CAD build for the part. Positions are in the model's coordinates, mm. A direction names the side the tool comes from. Coordinates: 2 decimals unless noted, no trailing zeros. Write each loop counter-clockwise with the first axis right and the second up, starting at its lowest first coordinate (ties: lowest second). Pieces come first, ordered by that corner, then holes. Notation, with made-up numbers: (64, 56.5) - (118, 56.5) arc R33 cw to (118, 91.5) - close; hole circle Ø1 at (-19.75, -8). An arc over 180 degrees is marked (long way). Answer in a Markdown table with one row per item. Add a question column.
Q1. Drill centre lines: line 1 along X through (y, z) = (21.5, -27); line 2 along Y through (x, z) = (36.5, 6.5); line 3 along Z through (x, y) = (14, 41). Where is each one in solid material? Low to high. Write a range as from..to.
Q2. Band-saw the part on B-B (y = 4.5). List the corners of the cut face in (x, z).
Q3. Band-saw the part on A-A (z = 5). List the corners of the cut face in (x, y).
Q4. Two-plate mould, pull along Z, no slides. Class faces 5 (the flat face through (-37.607, 3, 3)), 6 (the flat face through (0, 21, -43)), 7 (the flat face through (37.393, 21, -17)): +Z half, -Z half, draft (parallel to the pull), parting line (faces both ways), or undercut.
Q5. Band-saw the part on C-C (z = -4). List the corners of the cut face in (x, y), and give its area (3 significant figures).
Q6. Pin check, flat tips, straight feed: pin 1 (1 mm diameter, centred on y = 32.5, z = -13, fed in from -X); pin 2 (1.6 mm diameter, centred on x = -36.5, y = 40.5, fed in from +Z); pin 3 (1.6 mm diameter, centred on x = 36, z = -8, fed in from +Y). Stop position of each tip, or through.
Q7. Band-saw the part on D-D (x = 4.5). List the corners of the cut face in (y, z).
Q8. 3-axis set-ups, long thin cutter, end or side, ignore diameter. For faces 1 (the flat face through (35.393, 21, -18)), 2 (the flat face through (-37, 40, -9.5)), 3 (the flat face through (38, 6, 2)), 4 (the flat face through (-37, 43.5, -3)): which of +Z, -Z, +X, -X, +Y, -Y reach the whole face in a straight line?
```python
from build123d import *

# Parameters (mm, degrees)
BOSS_EXTRUDE1_DEPTH = 43.5
FILLET1_R           = 8
FILLET2_R           = 10
SKETCH3_W           = 3.5
SKETCH3_H           = 6
CUT_EXTRUDE1_DEPTH  = 57.75
BOSS_EXTRUDE2_DEPTH = 6


with BuildPart() as part:
    # Sketch2 → Boss-Extrude1 (new body)
    with BuildSketch(Plane(origin=(0, 0, 0), x_dir=(1, 0, 0), z_dir=(0, 1, 0))):
        Polygon((35.39315693, 0), (37.39315693, 0), (37.39315693, 45), (-37.60684307, 45), (-37.60684307, 0), (-35.60684307, 0), (-35.60684307, 43), (35.39315693, 43), align=None)
    extrude(amount=BOSS_EXTRUDE1_DEPTH)

    # Fillet1
    fillet1_edges = [part.edges().sort_by_distance(p)[0] for p in [
        (35.39315693, 21.75, -43),
        (-35.60684307, 21.75, -43),
    ]]
    fillet(fillet1_edges, radius=FILLET1_R)

    # Fillet2
    fillet2_edges = [part.edges().sort_by_distance(p)[0] for p in [
        (-37.60684307, 21.75, -45),
        (37.39315693, 21.75, -45),
    ]]
    fillet(fillet2_edges, radius=FILLET2_R)

    # Sketch3 → Cut-Extrude1 (cut, symmetric)
    with BuildSketch(Plane(origin=(0, 0, 0), x_dir=(0, 0, -1), z_dir=(1, 0, 0))):
        with Locations((7.75, 40.5)):
            Rectangle(SKETCH3_W, SKETCH3_H)
    extrude(amount=CUT_EXTRUDE1_DEPTH, both=True, mode=Mode.SUBTRACT)

    # Sketch4 → Boss-Extrude2 (add)
    with BuildSketch(Plane.XZ):
        Polygon((-37.60684307, -7), (-37.60684307, 6), (-35.60684307, 6), (-35.60684307, 7), (-37.60684307, 9), (-39.60684307, 9), (-39.60684307, -7), (-37.60684307, -9.5), align=None)
        Polygon((37.39315693, -7), (37.39315693, 6), (35.39315693, 6), (35.39315693, 7), (37.39315693, 9), (39.39315693, 9), (39.39315693, -7), (37.39315693, -9.5), align=None)
    extrude(amount=-BOSS_EXTRUDE2_DEPTH)


solid = part.part
```
Checked values:
| question | item | result |
|---|---|---|
| 1 | line 1 | x = -37.61..-35.61, 35.39..37.39 |
| 1 | line 2 | y = 0..6 |
| 1 | line 3 | z = -45..-43 |
| 2 | outline | (-39.61, -7) - (-37.61, -9.5) - (-37.61, -35) arc R10 ccw to (-27.61, -45) - (27.39, -45) arc R10 ccw to (37.39, -35) - (37.39, -9.5) - (39.39, -7) - (39.39, 9) - (37.39, 9) - (35.39, 7) - (35.39, 6) - (37.39, 6) - (37.39, 0) - (35.39, 0) - (35.39, -35) arc R8 cw to (27.39, -43) - (-27.61, -43) arc R8 cw to (-35.61, -35) - (-35.61, 0) - (-37.61, 0) - (-37.61, 6) - (-35.61, 6) - (-35.61, 7) - (-37.61, 9) - (-39.61, 9) - close |
| 3 | outline | (-39.61, 0) - (-37.61, 0) - (-37.61, 6) - (-39.61, 6) - close; (37.39, 0) - (39.39, 0) - (39.39, 6) - (37.39, 6) - close |
| 4 | face 5 | undercut |
| 4 | face 6 | +Z half |
| 4 | face 7 | draft |
| 5 | outline | (-39.61, 0) - (-35.61, 0) - (-35.61, 43.5) - (-37.61, 43.5) - (-37.61, 6) - (-39.61, 6) - close; (35.39, 0) - (39.39, 0) - (39.39, 6) - (37.39, 6) - (37.39, 43.5) - (35.39, 43.5) - close |
| 5 | area | 198 mm² |
| 6 | pin 1 | stops at x = -37.61 |
| 6 | pin 2 | stops at z = 0 |
| 6 | pin 3 | stops at y = 37.5 |
| 7 | outline | (0, -45) - (43.5, -45) - (43.5, -43) - (0, -43) - close |
| 8 | face 1 | +Z, +Y, -Y |
| 8 | face 2 | +X, -X, +Y |
| 8 | face 3 | +Z, +X, +Y |
| 8 | face 4 | +Z, -Z, +X, -X, +Y |
